Read the model definition and answer for the solid it produces. Units are mm, in the model's axes. Face numbers are marked on the shaded views. A direction names the side the tool comes from. Give positions to 0.01 mm unless a question says otherwise; leave off trailing zeros. Order: outer loops, then holes, each group sorted by start corner. A loop starts at its lowest first (then second) coordinate and runs counter-clockwise, first axis right, second up.
Item 1: Given pin 1 Ø10 at (x, z) = (0, 7) entering from +Y, flat-ended and moving along its own axis, determine where the tip first touches the part or whether it passes through.
Item 2: Find the intervals of material crossed by line 1 along Z through (x, y) = (-35.5, 10); line 2 along Y through (x, z) = (-39, 0.25), in increasing order.
Item 3: Which of the six approach directions +Z, -Z, +X, -X, +Y, -Y give full straight-line access (tool end or side, diameter ignored) to the marked faces 1 and 2?
Item 4: A cutting plane is placed at C-C (y = 10). Write down the section's boundary in (x, z), plus the area to 3 significant figures.
Item 5: A cutting plane is placed at A-A (x = -47). Write down the section's boundary in (y, z).
Item 6: A cutting plane is placed at B-B (z = 1.75). Write down the section's boundary in (x, y).
from build123d import *

# Parameters (mm, degrees)
F0_W     = 25.4
F0_H     = 25.4
F1_DEPTH = 63.5
F2_W     = 5.08
F2_H     = 12.7
F3_DEPTH = 127.001


with BuildPart() as f1:
    # F0 (on Right) → F1 (new body, symmetric)
    with BuildSketch(Plane.YZ):
        Rectangle(F0_W, F0_H)
    extrude(amount=F1_DEPTH, both=True)

    # F2 (on face) → F3 (cut, through all)
    with BuildSketch(Plane.YZ.offset(63.5)):
        with Locations((10.16, 6.35)):
            Rectangle(F2_W, F2_H)
    extrude(amount=-F3_DEPTH, mode=Mode.SUBTRACT)


solid = f1.part
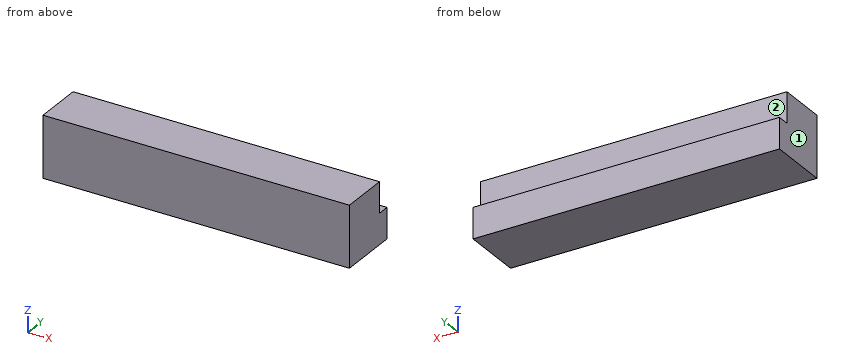
Response values:
1. pin 1: stops at y = 7.62
2. line 1: z = -12.7 to 0
2. line 2: y = -12.7 to 7.62
3. face 1: +Z, -Z, -X, +Y, -Y
3. face 2: +Z, +X, -X, +Y
4. outline: (-63.5, -12.7) - (63.5, -12.7) - (63.5, 0) - (-63.5, 0) - close
4. area: 1,610 mm2
5. outline: (-12.7, -12.7) - (12.7, -12.7) - (12.7, 0) - (7.62, 0) - (7.62, 12.7) - (-12.7, 12.7) - close
6. outline: (-63.5, -12.7) - (63.5, -12.7) - (63.5, 7.62) - (-63.5, 7.62) - close
